The figure shows three views and two pictorial views of one solid part (mm, origin at its lowest corner). Answer the questions. A direction names the side the tool comes from. Round coordinates to 2 decimals unless told otherwise and drop trailing zeros. Order: outer loops, then holes, each group sorted by start corner. A loop starts at its lowest first (then second) coordinate and runs counter-clockwise, first axis right, second up. Notation, with made-up numbers: (69, 73) -> (78, 73) arc R14 ccw to (78, 93) -> close; hole circle Ø7 at (57.5, 88). An arc over 180 degrees is marked (long way). Return JSON: item names as keys, results as strings. Group by question number.
(1) The part is cut by section C-C (x = 8.5). Determine the outline of the cut face in (y, z), plus the area to 3 significant figures.
(2) The part is cut by section B-B (y = 0.4). Determine the outline of the cut face in (x, z), plus the area to 3 significant figures.
(3) Consider line 1 (Z direction, x = 8.75, y = 1.5); line 2 (Z direction, x = 3.5, y = 0.4). Determine where each line is inside the solid, lowest interval first. Write a range as [from, to].
(4) Which of the six approach directions +Z, -Z, +X, -X, +Y, -Y give full straight-line access (tool end or side, diameter ignored) to the marked faces 1 and 2?
(5) The part is cut by section A-A (z = 8). Determine the outline of the cut face in (x, y).
(6) Determine the mould class of the marked faces 3, 4 and 5 for opening direction X: +X half, -X half, draft (parallel to the pull), parting line (faces both ways), or undercut.
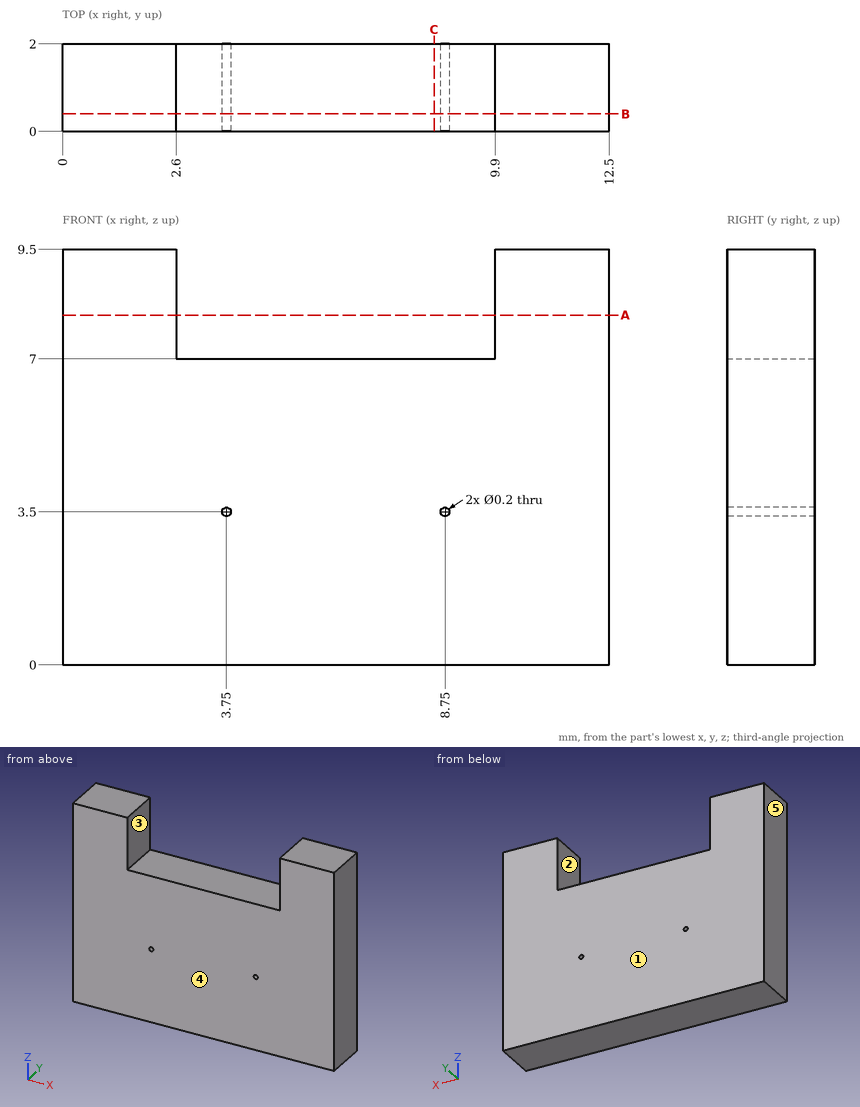
Answer below:
{
 "1": {"outline": "(0, 0) -> (2, 0) -> (2, 7) -> (0, 7) -> close", "area": "14.0 mm²"},
 "2": {"outline": "(0, 0) -> (12.5, 0) -> (12.5, 9.5) -> (9.9, 9.5) -> (9.9, 7) -> (2.6, 7) -> (2.6, 9.5) -> (0, 9.5) -> close; hole circle Ø0.2 at (3.75, 3.5); hole circle Ø0.2 at (8.75, 3.5)", "area": "100 mm²"},
 "3": {"line 1": "z = [0, 3.4], [3.6, 7]", "line 2": "z = [0, 7]"},
 "4": {"face 1": "+Z, -Z, +X, -X, +Y", "face 2": "+Z, +Y, -Y"},
 "5": {"outline": "(0, 0) -> (2.6, 0) -> (2.6, 2) -> (0, 2) -> close; (9.9, 0) -> (12.5, 0) -> (12.5, 2) -> (9.9, 2) -> close"},
 "6": {"face 3": "undercut", "face 4": "draft", "face 5": "-X half"}
}
